from build123d import *

# Parameters (mm, degrees)
SKETCH1_W           = 70
SKETCH1_H           = 50
BOSS_EXTRUDE1_DEPTH = 3
SKETCH2_W           = 3
SKETCH2_H           = 50
BOSS_EXTRUDE2_DEPTH = 60
SKETCH3_R           = 13.25
SKETCH3_R_2         = 2
CUT_EXTRUDE1_DEPTH  = 60
FILLET1_R           = 15
FILLET2_R           = 3


with BuildPart() as part:
    # Sketch1 → Boss-Extrude1 (new body)
    with BuildSketch(Plane(origin=(0, 0, 0), x_dir=(1, 0, 0), z_dir=(0, 1, 0))):
        with Locations((35, 25)):
            Rectangle(SKETCH1_W, SKETCH1_H)
        with BuildLine():
            Line((14, 45), (22, 45))
            ThreePointArc((22, 45), (24, 43), (22, 41))
            Line((22, 41), (14, 41))
            ThreePointArc((14, 41), (12, 43), (14, 45))
        make_face(mode=Mode.SUBTRACT)
        with BuildLine():
            Line((51, 45), (59, 45))
            ThreePointArc((59, 45), (61, 43), (59, 41))
            Line((59, 41), (51, 41))
            ThreePointArc((51, 41), (49, 43), (51, 45))
        make_face(mode=Mode.SUBTRACT)
        with BuildLine():
            Line((51, 5), (59, 5))
            ThreePointArc((59, 5), (61, 7), (59, 9))
            Line((59, 9), (51, 9))
            ThreePointArc((51, 9), (49, 7), (51, 5))
        make_face(mode=Mode.SUBTRACT)
        with BuildLine():
            Line((14, 5), (22, 5))
            ThreePointArc((22, 5), (24, 7), (22, 9))
            Line((22, 9), (14, 9))
            ThreePointArc((14, 9), (12, 7), (14, 5))
        make_face(mode=Mode.SUBTRACT)
    extrude(amount=BOSS_EXTRUDE1_DEPTH)

    # Sketch2 → Boss-Extrude2 (add)
    with BuildSketch(Plane(origin=(0, 3, 0), x_dir=(1, 0, 0), z_dir=(0, 1, 0))):
        with Locations((1.5, 25)):
            Rectangle(SKETCH2_W, SKETCH2_H)
    extrude(amount=BOSS_EXTRUDE2_DEPTH)

    # Sketch3 → Cut-Extrude1 (cut)
    with BuildSketch(Plane.ZY):
        with Locations((-25, 38.75)):
            Circle(SKETCH3_R)
        with Locations((-12.625631329, 26.375631329)):
            Circle(SKETCH3_R_2)
        with Locations((-12.625631329, 51.124368671)):
            Circle(SKETCH3_R_2)
        with Locations((-37.374368671, 51.124368671)):
            Circle(SKETCH3_R_2)
        with Locations((-37.374368671, 26.375631329)):
            Circle(SKETCH3_R_2)
    extrude(amount=-CUT_EXTRUDE1_DEPTH, mode=Mode.SUBTRACT)

    # Fillet1
    fillet1_edges = [part.edges().sort_by_distance(p)[0] for p in [
        (1.5, 63, 0),
        (1.5, 63, -50),
    ]]
    fillet(fillet1_edges, radius=FILLET1_R)

    # Fillet2
    fillet2_edges = [part.edges().sort_by_distance(p)[0] for p in [
        (0, 0, -25),
        (70, 1.5, -50),
        (70, 1.5, 0),
    ]]
    fillet(fillet2_edges, radius=FILLET2_R)


solid = part.part
Build history of the part. All positions in model axes, mm. A direction names the side the tool comes from. Give positions to 0.01 mm unless a question says otherwise; leave off trailing zeros. Order: outer loops, then holes, each group sorted by start corner. A loop starts at its lowest first (then second) coordinate and runs counter-clockwise, first axis right, second up. Notation, with made-up numbers: M 39.5,37.25 L 75.5,37.25 A19 cw 75.5,56.25 Z; hole C 65,89 d7. An arc over 180 degrees is marked long. Put each result on its own line as item: value.
Item 1: Flat gauge pins, fed straight in: pin 1 Ø2 at (x, z) = (35, -17.5) entering from +Y; pin 2 Ø4 at (y, z) = (48.5, -9) entering from +X. Where does each tip first touch, or does it go through?
From the geometry:
pin 1: stops at y = 3
pin 2: stops at x = 3
Item 2: Slice it at A-A, the plane z = -25. Write the cut outline in (x, y), plus the area to 3 significant figures.
From the geometry:
outline: M 0,3 A3 ccw 3,0 L 70,0 L 70,3 L 3,3 L 3,25.5 L 0,25.5 Z; M 0,52 L 3,52 L 3,63 L 0,63 Z
area: 309 mm2
Item 3: Slice it at D-D, the plane z = -43. Write the cut outline in (x, y), plus the area to 3 significant figures.
From the geometry:
outline: M 0,3 A3 ccw 3,0 L 12,0 L 12,3 L 3,3 L 3,60.69 L 0,60.69 Z; M 24,0 L 49,0 L 49,3 L 24,3 Z; M 61,0 L 70,0 L 70,3 L 61,3 Z
area: 309 mm2
Item 4: Probe line 1 (X direction, y = 5.5, z = -36.5). List the from-to ranges inside material, lowest first. Write a range as [from, to].
From the geometry:
line 1: x = [0, 3]
Item 5: Two-plate mould, pull along X, no slides. Class faces 1 (the cylindrical face through (1.479, 50.358, -10.778)), 2 (the cylindrical face through (69.1, 1.52, -49.14)), 3 (the flat face through (55, 1, -41)): +X half, -X half, draft (parallel to the pull), parting line (faces both ways), or undercut.
From the geometry:
face 1: draft
face 2: +X half
face 3: undercut
Item 6: Slice it at B-B, the plane y = 38.75. Write the cut outline in (x, z), plus the area to 3 significant figures.
From the geometry:
outline: M 0,-50 L 3,-50 L 3,-38.25 L 0,-38.25 Z; M 0,-11.75 L 3,-11.75 L 3,0 L 0,0 Z
area: 70.5 mm2
Item 7: 3-axis set-ups, long thin cutter, end or side, ignore diameter. For faces 4 (the flat face through (3, 26, -19)), 5 (the cylindrical face through (12, 1, -43)), 6 (the flat face through (23.4, 2.6, 0)): which of +Z, -Z, +X, -X, +Y, -Y reach the whole face in a straight line?
From the geometry:
face 4: +Z, -Z, +X, +Y
face 5: +Y, -Y
face 6: +Z, +X, -X, +Y, -Y
Item 8: Slice it at C-C, the plane x = 56.5. Write the cut outline in (y, z), plus the area to 3 significant figures.
From the geometry:
outline: M 0,-50 L 3,-50 L 3,-45 L 0,-45 Z; M 0,-41 L 3,-41 L 3,-9 L 0,-9 Z; M 0,-5 L 3,-5 L 3,0 L 0,0 Z
area: 126 mm2
